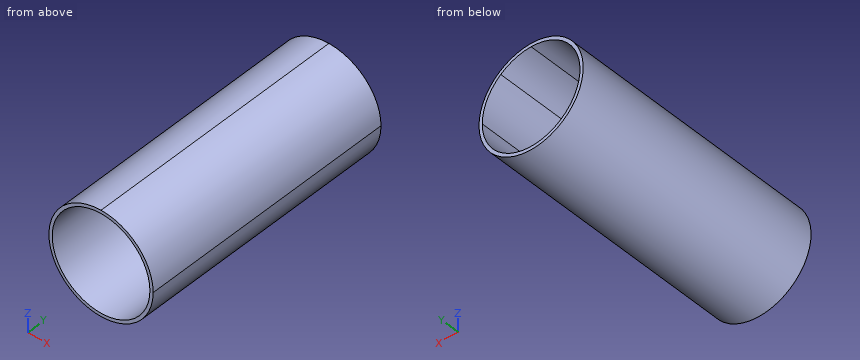
from build123d import *

# Parameters (mm, degrees)
F1_DEPTH = 400


with BuildPart() as f1:
    # F0 (on Front) → F1 (new body)
    with BuildSketch(Plane.XZ):
        with BuildLine():
            ThreePointArc((0, 80), (-56.568542, -56.568542), (80, 0))
            ThreePointArc((80, 0), (56.568542, 56.568542), (0, 80))
        make_face()
        with BuildLine():
            ThreePointArc((75, 0), (-53.033009, -53.033009), (0, 75))
            ThreePointArc((0, 75), (24.670108, 70.826448), (46.594564, 58.770287))
            ThreePointArc((46.594564, 58.770287), (67.526263, 32.637461), (75, 0))
        make_face(mode=Mode.SUBTRACT)
    extrude(amount=F1_DEPTH)


solid = f1.part
The model under review builds one solid part; all positions refer to its coordinate system, in mm. Round coordinates to 2 decimals unless told otherwise and drop trailing zeros. Write each loop counter-clockwise with the first axis right and the second up, starting at its lowest first coordinate (ties: lowest second). Pieces come first, ordered by that corner, then holes. Notation, with made-up numbers: M 86.5,33 L 103.5,33 A21 ccw 103.5,56 Z; hole C 64,-10.75 d1. An arc over 180 degrees is marked long. Answer as CSV lines item,"result". Start each with the question number.
Q1. Wall thickness on line 1 along Z through (x, y) = (49, -273.5); line 2 along Z through (x, y) = (32.5, -222); line 3 along X through (y, z) = (-318, 66.5): over which ranges is each line inside the solid? List them lowest first.
Q2. Consider section A-A, the plane x = -33. Give the boundary of the cut face in (y, z).
Q3. Consider section C-C, the plane y = -349.5. Give the boundary of the cut face in (x, z), then the cut area to 3 significant figures.
Q4. Clearance check with flat-ended pins moving along their axes: P1, Ø2, axis at x = -5, y = -237, coming from the +Z side; P2, Ø4, axis at x = 10, y = -348.5, coming from the +Z side; P3, Ø2, axis at x = 54.5, y = -82.5, coming from the -Z side. State where each tip first meets the part, or that it passes through.
Q5. Consider section B-B, the plane z = 28.5. Give the boundary of the cut face in (x, y).
Result set:
1,line 1,"z = -63.24 to -56.78, 56.78 to 63.24"
1,line 2,"z = -73.1 to -67.59, 67.59 to 73.1"
1,line 3,"x = -44.47 to -34.68, 34.68 to 44.47"
2,outline,"M -400,-72.88 L 0,-72.88 L 0,-67.35 L -400,-67.35 Z; M -400,67.35 L 0,67.35 L 0,72.88 L -400,72.88 Z"
3,outline,"M 0,80 A80 ccw long 80,0 A80 ccw Z; hole M 0,75 A75 ccw long 75,0 A75 ccw 46.59,58.77 A75 ccw Z"
3,area,"2,430 mm²"
4,P1,"stops at z = 79.9"
4,P2,"stops at z = 79.6"
4,P3,"stops at z = -59.48"
5,outline,"M -74.75,-400 L -69.37,-400 L -69.37,0 L -74.75,0 Z; M 69.37,-400 L 74.75,-400 L 74.75,0 L 69.37,0 Z"
